```python
from build123d import *

# Parameters (mm, degrees)
SKETCH1_W           = 325
SKETCH1_H           = 245
BOSS_EXTRUDE1_DEPTH = 10
SKETCH2_W           = 325
SKETCH2_H           = 245
SKETCH2_W_2         = 291
SKETCH2_H_2         = 211
BOSS_EXTRUDE2_DEPTH = 49.8
SKETCH3_W           = 325
SKETCH3_H           = 245
SKETCH3_W_2         = 305
SKETCH3_H_2         = 225
BOSS_EXTRUDE3_DEPTH = 10
SKETCH4_R           = 15
CUT_EXTRUDE1_DEPTH  = 30
CHAMFER1_SIZE       = 10
SKETCH5_W           = 24
SKETCH5_H           = 10
CUT_EXTRUDE2_DEPTH  = 289.552057695
SKETCH6_W           = 33.4
SKETCH6_H           = 10
CUT_EXTRUDE3_DEPTH  = 10


with BuildPart() as part:
    # Sketch1 → Boss-Extrude1 (new body)
    with BuildSketch(Plane(origin=(0, 0, 0), x_dir=(1, 0, 0), z_dir=(0, 1, 0))):
        Rectangle(SKETCH1_W, SKETCH1_H)
    extrude(amount=BOSS_EXTRUDE1_DEPTH)

    # Sketch2 → Boss-Extrude2 (add)
    with BuildSketch(Plane(origin=(0, 10, 0), x_dir=(1, 0, 0), z_dir=(0, 1, 0))):
        Rectangle(SKETCH2_W, SKETCH2_H)
        Rectangle(SKETCH2_W_2, SKETCH2_H_2, mode=Mode.SUBTRACT)
    extrude(amount=BOSS_EXTRUDE2_DEPTH)

    # Sketch3 → Boss-Extrude3 (add)
    with BuildSketch(Plane(origin=(0, 59.8, 0), x_dir=(1, 0, 0), z_dir=(0, 1, 0))):
        Rectangle(SKETCH3_W, SKETCH3_H)
        Rectangle(SKETCH3_W_2, SKETCH3_H_2, mode=Mode.SUBTRACT)
    extrude(amount=BOSS_EXTRUDE3_DEPTH)

    # Sketch4 → Cut-Extrude1 (cut)
    with BuildSketch(Plane.ZY.offset(162.5)):
        with Locations((0, 34.9)):
            Circle(SKETCH4_R)
    extrude(amount=-CUT_EXTRUDE1_DEPTH, mode=Mode.SUBTRACT)

    # Chamfer1
    chamfer1_edges = [part.edges().sort_by_distance(p)[0] for p in [
        (-162.5, 34.9, -15),
    ]]
    chamfer(chamfer1_edges, length=CHAMFER1_SIZE)

    # Sketch5 → Cut-Extrude2 (cut, through all)
    with BuildSketch(Plane.XY.offset(-105.5)):
        with Locations((1.5, 20)):
            Rectangle(SKETCH5_W, SKETCH5_H)
    extrude(amount=-CUT_EXTRUDE2_DEPTH, mode=Mode.SUBTRACT)

    # Sketch6 → Cut-Extrude3 (cut)
    with BuildSketch(Plane.XY.offset(-105.5)):
        with Locations((1.5, 20)):
            Rectangle(SKETCH6_W, SKETCH6_H)
    extrude(amount=-CUT_EXTRUDE3_DEPTH, mode=Mode.SUBTRACT)


solid = part.part
```
Work out the finished part from the listing and answer in its coordinate system (mm). A direction names the side the tool comes from. Give positions to 0.01 mm unless a question says otherwise; leave off trailing zeros. Loops run counter-clockwise (first coordinate to the right, second up) from the corner with the lowest first, then second, coordinate; pieces in that order, holes last. Notation, with made-up numbers: (53.25, 25.5) - (59.25, 25.5) arc R23 ccw to (59.25, 33.5) - close; hole circle Ø2 at (86.5, 50.25). An arc over 180 degrees is marked (long way). Use CSV: the item, a comma, the result in double quotes. Start each with the question number.
(1) Find section B-B, the plane x = -4. Determine the outline of the cut face in (y, z).
(2) Determine the mould class of faces 1 (the face through (-149.049, 20.257, -3.252)), 2 (the face through (-2, 0, -2)), 3 (the face through (1, 15, -114)) for opening direction Z: released by +Z, released by -Z, zero draft, split by the parting line, or undercut.
(3) A tool of negligible diameter and unlimited length cuts with its end or side. For faces 4 (the face through (13.5, 20, -119)), 5 (the face through (-2, 65, 112.5)), 6 (the face through (18.2, 20, -110)), from which of +Z, -Z, +X, -X, +Y, -Y can it reach the whole face along a straight path? Write none if from no direction.
(4) Find the intervals of material crossed by L1, parallel to Y at x = -148, z = 0; L2, parallel to Z at x = -133, y = 57; L3, parallel to X at y = 50, z = -52.5, in increasing order.
(5) Find section D-D, the plane z = -75.5. Determine the outline of the cut face in (x, y).
(6) Each of these flat-tipped pins is pushed along its axis until it touches: pin 1 (1 mm diameter, centred on x = -74.5, z = 12, fed in from +Y); pin 2 (24 mm diameter, centred on y = 34.9, z = 0, fed in from -X). Where does it stop, or does it pass through?
(7) Find section A-A, the plane z = 0. Determine the outline of the cut face in (x, y).
(8) Find section C-C, the plane y = 34.9. Determine the outline of the cut face in (x, z).
Results found:
1,outline,"(0, -122.5) - (15, -122.5) - (15, -105.5) - (10, -105.5) - (10, 105.5) - (59.8, 105.5) - (59.8, 112.5) - (69.8, 112.5) - (69.8, 122.5) - (0, 122.5) - close; (25, -122.5) - (69.8, -122.5) - (69.8, -112.5) - (59.8, -112.5) - (59.8, -105.5) - (25, -105.5) - close"
2,face 1,"undercut"
2,face 2,"zero draft"
2,face 3,"undercut"
3,face 4,"-Z"
3,face 5,"+Y"
3,face 6,"none"
4,L1,"0 to 19.9, 49.9 to 59.8"
4,L2,"-122.5 to -105.5, 105.5 to 122.5"
4,L3,"-162.5 to -145.5, 145.5 to 162.5"
5,outline,"(-162.5, 0) - (162.5, 0) - (162.5, 69.8) - (152.5, 69.8) - (152.5, 59.8) - (145.5, 59.8) - (145.5, 10) - (-145.5, 10) - (-145.5, 59.8) - (-152.5, 59.8) - (-152.5, 69.8) - (-162.5, 69.8) - close"
6,pin 1,"y = 10"
6,pin 2,"x = 145.5"
7,outline,"(-162.5, 0) - (162.5, 0) - (162.5, 69.8) - (152.5, 69.8) - (152.5, 59.8) - (145.5, 59.8) - (145.5, 10) - (-145.5, 10) - (-145.5, 19.9) - (-152.5, 19.9) - (-162.5, 9.9) - close; (-162.5, 59.9) - (-152.5, 49.9) - (-145.5, 49.9) - (-145.5, 59.8) - (-152.5, 59.8) - (-152.5, 69.8) - (-162.5, 69.8) - close"
8,outline,"(-162.5, -122.5) - (162.5, -122.5) - (162.5, 122.5) - (-162.5, 122.5) - (-162.5, 25) - (-152.5, 15) - (-145.5, 15) - (-145.5, 105.5) - (145.5, 105.5) - (145.5, -105.5) - (-145.5, -105.5) - (-145.5, -15) - (-152.5, -15) - (-162.5, -25) - close"
